Source: three-view drawing plus pictorial views. Frame: mm from the lowest corner of the part. Coordinates: 2 decimals unless noted, no trailing zeros. Order: outer loops, then holes, each group sorted by start corner. A loop starts at its lowest first (then second) coordinate and runs counter-clockwise, first axis right, second up. Notation, with made-up numbers: (-37, 59) - (-11, 59) arc R22 ccw to (-11, 80) - close; hole circle Ø1 at (81, 36). An arc over 180 degrees is marked (long way). One line per question, with ' | ' between items.
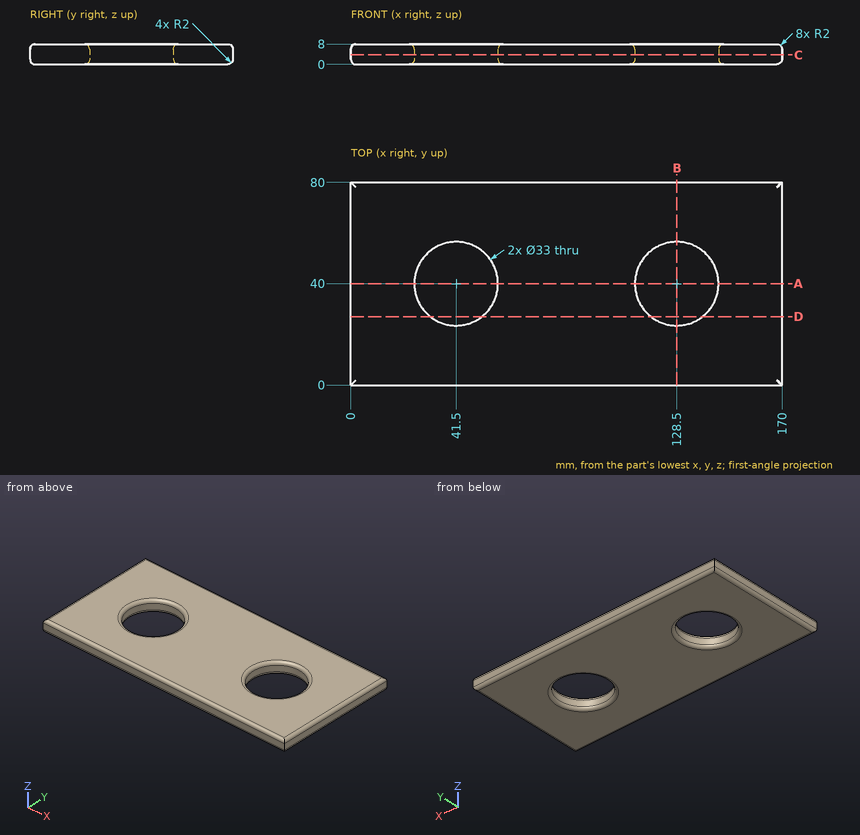
Item 1: Section D-D on y = 27. Count the separate pieces of the cut face and the enclosed holes in it, and give its area (3 significant figures).
Data:
separate pieces: 3 | enclosed holes: 0 | area: 1,020 mm^2
Item 2: Section C-C on z = 3.75. Return the cut outline in (x, y).
Data:
outline: (0, 0) - (170, 0) - (170, 80) - (0, 80) - close; hole circle Ø33 at (41.5, 40); hole circle Ø33 at (128.5, 40)
Item 3: Section A-A on y = 40. Return the cut outline in (x, z), and give its area (3 significant figures).
Data:
outline: (0, 2) arc R2 ccw to (2, 0) - (23, 0) arc R2 ccw to (25, 2) - (25, 6) arc R2 ccw to (23, 8) - (2, 8) arc R2 ccw to (0, 6) - close; (58, 2) arc R2 ccw to (60, 0) - (110, 0) arc R2 ccw to (112, 2) - (112, 6) arc R2 ccw to (110, 8) - (60, 8) arc R2 ccw to (58, 6) - close; (145, 2) arc R2 ccw to (147, 0) - (168, 0) arc R2 ccw to (170, 2) - (170, 6) arc R2 ccw to (168, 8) - (147, 8) arc R2 ccw to (145, 6) - close | area: 822 mm^2
Item 4: Contact query for a flat-ended pin moving along its axis: P1, Ø1, axis at x = 98.5, z = 7, coming from the -Y side. Output: stop coordinate, or through.
Data:
P1: y = 0.06
Item 5: Ray query, line 1 (Y direction, x = 41.5, z = 4.25); line 2 (Y direction, x = 120, z = 1.25); line 3 (X direction, y = 12.5, z = 1.25). Return the intervals inside material, ascending.
Data:
line 1: 0 to 23.5, 56.5 to 80 | line 2: 0.15 to 25.69, 54.31 to 79.85 | line 3: 0.15 to 169.85
Item 6: Section B-B on x = 128.5. Return the cut outline in (y, z), and give its area (3 significant figures).
Data:
outline: (0, 2) arc R2 ccw to (2, 0) - (21.5, 0) arc R2 ccw to (23.5, 2) - (23.5, 6) arc R2 ccw to (21.5, 8) - (2, 8) arc R2 ccw to (0, 6) - close; (56.5, 2) arc R2 ccw to (58.5, 0) - (78, 0) arc R2 ccw to (80, 2) - (80, 6) arc R2 ccw to (78, 8) - (58.5, 8) arc R2 ccw to (56.5, 6) - close | area: 369 mm^2
